Here's how the part is built. I have some questions about the finished solid (model axes, mm). Face numbers are marked on the shaded views. A direction names the side the tool comes from. Coordinates: 2 decimals unless noted, no trailing zeros. Write each loop counter-clockwise with the first axis right and the second up, starting at its lowest first coordinate (ties: lowest second). Pieces come first, ordered by that corner, then holes. Notation, with made-up numbers: (22, 80.25) -> (62, 80.25) arc R31 cw to (62, 116.25) -> close; hole circle Ø8 at (45.25, 53.5). An arc over 180 degrees is marked (long way). Answer in a Markdown table with one row per item. Add a question column.
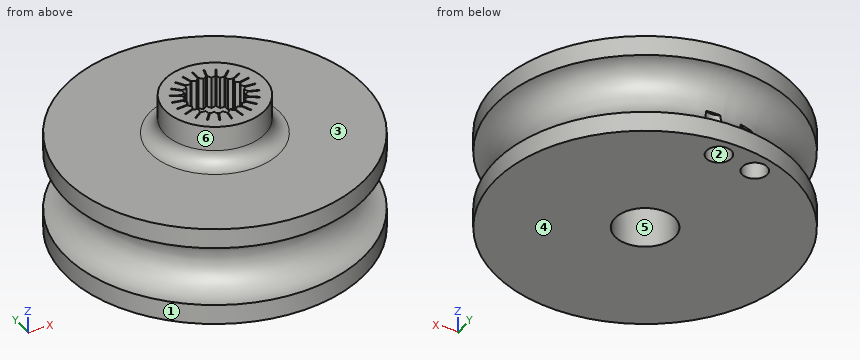
from build123d import *

# Parameters (mm, degrees)
SKETCH_6_R          = 5
EXTRUDE_3_DEPTH     = 4
CUT_EXTRUDE_START   = 4
CUT_EXTRUDE_5_DEPTH = 3.2
FILLET_2_R          = 1.5
SKETCH_9_R          = 1.9
CUT_EXTRUDE_6_DEPTH = 26.416530054
SKETCH_10_R         = 3
CUT_EXTRUDE_7_DEPTH = 5.8
SKETCH_11_R         = 1.25
CUT_EXTRUDE_8_DEPTH = 5


with BuildPart() as part:
    # ｽｹｯﾁ8 → 回転1 (revolve)
    with BuildSketch(Plane(origin=(0, 0, 0), x_dir=(1, 0, 0), z_dir=(0, 1, 0))):
        with BuildLine():
            Line((0, 0), (0, 10))
            Line((0, 10), (15, 10))
            Line((15, 10), (15, 8))
            ThreePointArc((15, 8), (12, 5), (15, 2))
            Line((15, 2), (15, 0))
            Line((15, 0), (0, 0))
        make_face()
    revolve(axis=Axis((0, 0, 0), (0, 0, -1)))

    # ｽｹｯﾁ6 → ﾎﾞｽ - 押し出し3 (add)
    with BuildSketch(Plane.XY):
        Circle(SKETCH_6_R)
    extrude(amount=EXTRUDE_3_DEPTH)

    # ｽｹｯﾁ5 → ｶｯﾄ - 押し出し5 (cut)
    with BuildSketch(Plane.XY.offset(CUT_EXTRUDE_START)):
        Polygon((-0.05, 2.95), (-0.05, 3.95), (0.05, 3.95), (0.05, 2.95), (0.362514094, 2.637485906), (0.747754611, 2.854095836), (1.017551382, 3.817013124), (1.11384311, 3.790033446), (0.844046339, 2.827116159), (1.060656269, 2.441875642), (1.490051682, 2.546516441), (2.009635632, 3.400935845), (2.095077573, 3.34897745), (1.575493623, 2.494558046), (1.680134421, 2.065162633), (2.121838437, 2.050073571), (2.852674402, 2.732626714), (2.920929716, 2.659543117), (2.190093752, 1.976989974), (2.17500469, 1.535285958), (2.596258142, 1.401586122), (3.484143361, 1.86165116), (3.530149865, 1.772862638), (2.642264646, 1.3127976), (2.50856481, 0.891544148), (2.878125258, 0.649149443), (3.857209346, 0.852605456), (3.877554947, 0.754697047), (2.898470859, 0.551241034), (2.656076155, 0.181680586), (2.94653499, -0.151431681), (3.944203759, -0.219674094), (3.937379518, -0.319440971), (2.939710748, -0.251198558), (2.606598481, -0.541657393), (2.796413701, -0.94078181), (3.738674623, -1.275661422), (3.705186662, -1.369887514), (2.76292574, -1.035007902), (2.363801323, -1.224823122), (2.4388952, -1.660358456), (3.255865093, -2.237038778), (3.198197061, -2.318735767), (2.381227168, -1.742055445), (1.945691834, -1.817149322), (1.900495, -2.25679391), (2.531582945, -3.032505201), (2.454011816, -3.095613995), (1.822923871, -2.319902705), (1.383279283, -2.274705871), (1.22114378, -2.685853285), (1.61954487, -3.603064586), (1.52782374, -3.642904695), (1.12942265, -2.725693394), (0.718275236, -2.563557891), (0.451225912, -2.915715208), (0.587392561, -3.906401154), (0.488323967, -3.920017819), (0.352157318, -2.929331873), (0, -2.66228255), (-0.352157318, -2.929331873), (-0.488323967, -3.920017819), (-0.587392561, -3.906401154), (-0.451225912, -2.915715208), (-0.718275236, -2.563557891), (-1.12942265, -2.725693394), (-1.52782374, -3.642904695), (-1.61954487, -3.603064586), (-1.22114378, -2.685853285), (-1.383279283, -2.274705871), (-1.822923871, -2.319902705), (-2.454011816, -3.095613995), (-2.531582945, -3.032505201), (-1.900495, -2.25679391), (-1.945691834, -1.817149322), (-2.381227168, -1.742055445), (-3.198197061, -2.318735767), (-3.255865093, -2.237038778), (-2.4388952, -1.660358456), (-2.363801323, -1.224823122), (-2.76292574, -1.035007902), (-3.705186662, -1.369887514), (-3.738674623, -1.275661422), (-2.796413701, -0.94078181), (-2.606598481, -0.541657393), (-2.939710748, -0.251198558), (-3.937379518, -0.319440971), (-3.944203759, -0.219674094), (-2.94653499, -0.151431681), (-2.656076155, 0.181680586), (-2.898470859, 0.551241034), (-3.877554947, 0.754697047), (-3.857209346, 0.852605456), (-2.878125258, 0.649149443), (-2.50856481, 0.891544148), (-2.642264646, 1.3127976), (-3.530149865, 1.772862638), (-3.484143361, 1.86165116), (-2.596258142, 1.401586122), (-2.17500469, 1.535285958), (-2.190093752, 1.976989974), (-2.920929716, 2.659543117), (-2.852674402, 2.732626714), (-2.121838437, 2.050073571), (-1.680134421, 2.065162633), (-1.575493623, 2.494558046), (-2.095077573, 3.34897745), (-2.009635632, 3.400935845), (-1.490051682, 2.546516441), (-1.060656269, 2.441875642), (-0.844046339, 2.827116159), (-1.11384311, 3.790033446), (-1.017551382, 3.817013124), (-0.747754611, 2.854095836), (-0.362514094, 2.637485906), align=None)
    extrude(amount=-CUT_EXTRUDE_5_DEPTH, mode=Mode.SUBTRACT)

    # ﾌｨﾚｯﾄ2
    fillet_2_edges = [part.edges().sort_by_distance(p)[0] for p in [
        (-5, 0, 0),
    ]]
    fillet(fillet_2_edges, radius=FILLET_2_R)

    # ｽｹｯﾁ9 → ｶｯﾄ - 押し出し6 (cut, through all)
    with BuildSketch(Plane(origin=(0, 0, -10), x_dir=(-1, 0, 0), z_dir=(0, 0, -1))):
        Circle(SKETCH_9_R)
    extrude(amount=-CUT_EXTRUDE_6_DEPTH, mode=Mode.SUBTRACT)

    # ｽｹｯﾁ10 → ｶｯﾄ - 押し出し7 (cut)
    with BuildSketch(Plane(origin=(0, 0, -10), x_dir=(-1, 0, 0), z_dir=(0, 0, -1))):
        Circle(SKETCH_10_R)
    extrude(amount=-CUT_EXTRUDE_7_DEPTH, mode=Mode.SUBTRACT)

    # ｽｹｯﾁ11 → ｶｯﾄ - 押し出し8 (cut)
    with BuildSketch(Plane.XY.offset(-10)):
        with Locations(Location((0, 13, 0), (0, 0, 234.816184512))):
            Circle(SKETCH_11_R)
        with Locations(Location((-3.952379255, 12.384615385, 0), (0, 0, 252.515950709))):
            Circle(SKETCH_11_R)
    extrude(amount=CUT_EXTRUDE_8_DEPTH, mode=Mode.SUBTRACT)


solid = part.part
Q1. Imagine slicing it at B-B on y = 13. State how many separate pieces and enclosed holes the cut face has, plus the area to 3 significant figures.
Q2. Imagine slicing it at A-A on z = -7.25. Please give me the cut outline in (x, y).
Q3. If we mould it in two halves opening along X, with no side actions, what happens to the marked faces 4, 5 and 6? For each: pulls with the +X half, pulls with the -X half, needs draft (parallel to the pull), parting line crosses it, or undercut.
Q4. I'm going to push flat-ended pins straight in: P1, Ø1.1, axis at y = 3.5, z = 3, coming from the +X side; P2, Ø3, axis at x = -3.95, y = 12.38, coming from the +Z side; P3, Ø5, axis at y = -5.5, z = 0.5, coming from the -X side. Where does each tip first touch, or does it pass through?
Q5. I need wall thicknesses on line 1 (Y direction, x = 0, z = -8.05); line 2 (Z direction, x = -11, y = 6); line 3 (Z direction, x = 7, y = 6.5). Which ranges of each line are inside material? Lowest first, please. Write a range as [from, to].
Q6. Imagine slicing it at C-C on z = -9. Please give me the cut outline in (x, y), plus the area to 3 significant figures.
Q7. For the marked faces 1, 2 and 3, which set-ups out of +Z, -Z, +X, -X, +Y, -Y let a thin tool reach every point of the face, with its end or its side?
Q8. Imagine slicing it at D-D on z = -0.75. Please give me the cut outline in (x, y).
Result sheet:
| question | item | result |
|---|---|---|
| 1 | separate pieces | 4 |
| 1 | enclosed holes | 0 |
| 1 | area | 59.4 mm^2 |
| 2 | outline | (-5.13, 11.96) arc R13.02 ccw (long way) to (1.25, 12.96) arc R1.25 cw to (-1.25, 12.96) arc R13.02 ccw to (-2.75, 12.72) arc R1.25 cw to start; hole circle Ø6 at (0, 0) |
| 3 | face 4 | needs draft |
| 3 | face 5 | undercut |
| 3 | face 6 | parting line crosses it |
| 4 | P1 | stops at x = 4.04 |
| 4 | P2 | stops at z = 0 |
| 4 | P3 | stops at x = -14.69 |
| 5 | line 1 | y = [-15, -3], [3, 11.75], [14.25, 15] |
| 5 | line 2 | z = [-10, -6.7], [-3.3, 0] |
| 5 | line 3 | z = [-10, 0] |
| 6 | outline | circle Ø30 at (0, 0); hole circle Ø2.5 at (-3.95, 12.38); hole circle Ø6 at (0, 0); hole circle Ø2.5 at (0, 13) |
| 6 | area | 669 mm^2 |
| 7 | face 1 | +Z, -Z |
| 7 | face 2 | -Z |
| 7 | face 3 | +Z |
| 8 | outline | circle Ø30 at (0, 0); hole circle Ø3.8 at (0, 0) |
